The figure shows three views and two pictorial views of one solid part (mm, origin at its lowest corner). Answer the questions. Coordinates: 2 decimals unless noted, no trailing zeros. Order: outer loops, then holes, each group sorted by start corner. A loop starts at its lowest first (then second) coordinate and runs counter-clockwise, first axis right, second up. Notation, with made-up numbers: (-28.75, 4) -> (-10.75, 4) arc R18 cw to (-10.75, 26) -> close; hole circle Ø10 at (-25, -6). An arc over 180 degrees is marked (long way). Write item = value, one per line. Start each with the question number.
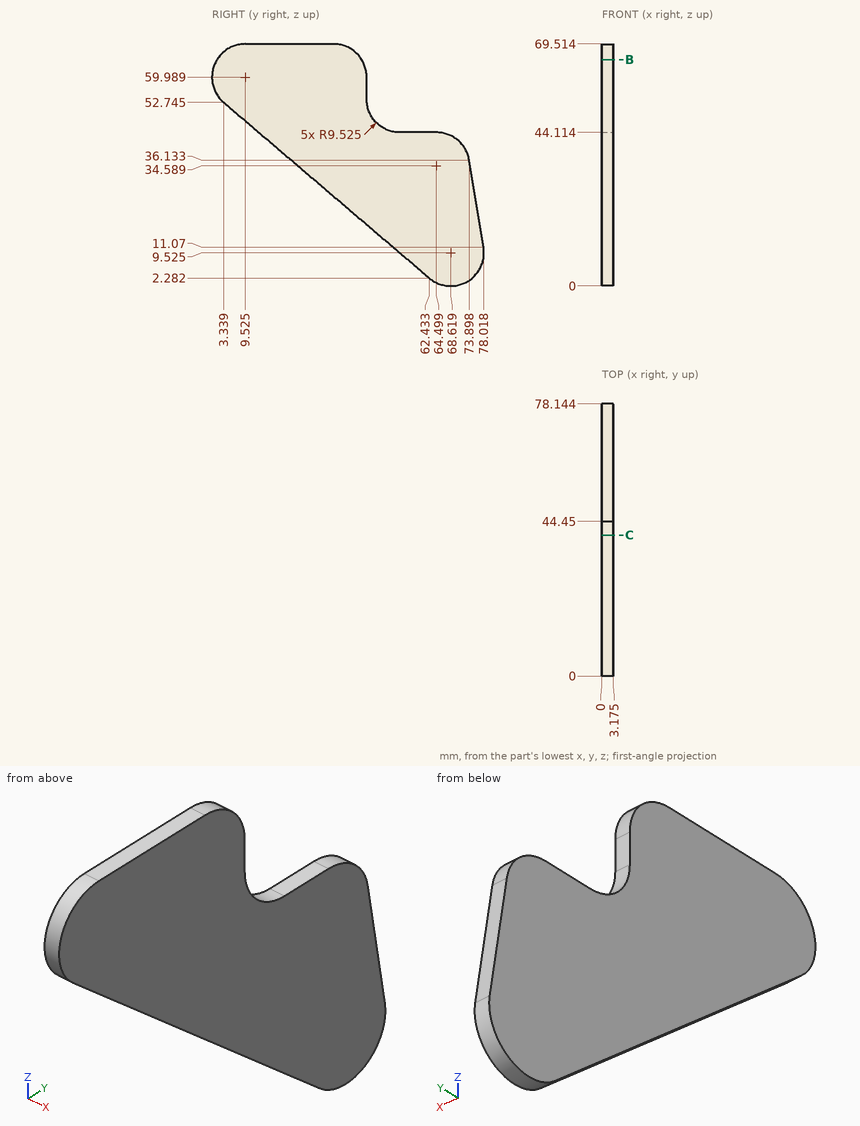
Item 1: Section B-B, the plane z = 65 is taken. Give the vertices of the cut face in (x, y) (1 decimal).
Item 2: Consider probe 1 along Y at (x, z) = (2.35, 30) (1 decimal); probe 2 along Z at (x, y) = (1.2, 22.5) (1 decimal); probe 3 along Y at (x, z) = (2.3, 9.5) (1 decimal). Determine where each line is inside the solid, lowest interval first.
Item 3: Section C-C, the plane y = 40.5 is taken. Give the vertices of the cut face in (x, z) (1 decimal).
Item 4: Each of these flat-tipped pins is pushed along its axis until it touches: pin 1 (1 mm diameter, centred on x = 1, y = 59.5, fed in from +Z); pin 2 (1 mm diameter, centred on x = 0.5, z = 37.5, fed in from -Y) (1 decimal). Where does it stop, or does it pass through?
A:
q1.outline = (0, 1.4) -> (3.2, 1.4) -> (3.2, 43) -> (0, 43) -> close
q2.probe_1 = 30 to 74.9
q2.probe_2 = 36.4 to 69.5
q2.probe_3 = 54 to 78.1
q3.outline = (0, 21) -> (3.2, 21) -> (3.2, 67.7) -> (0, 67.7) -> close
q4.pin_1 = 44.11
q4.pin_2 = 20.6
